Geometry: final body of the model. Coordinates: model frame, mm. A direction names the side the tool comes from. Give positions to 0.01 mm unless a question says otherwise; leave off trailing zeros. Loops run counter-clockwise (first coordinate to the right, second up) from the corner with the lowest first, then second, coordinate; pieces in that order, holes last. Notation, with made-up numbers: (-7.75, -30) -> (51.25, -30) arc R26 ccw to (51.25, -8) -> close; hole circle Ø8 at (-35, 80). An arc over 180 degrees is marked (long way). Answer in a Markdown table with one row per item. Add a question column.
from build123d import *

# Parameters (mm, degrees)
SKETCH1_W               = 50.8
SKETCH1_H               = 25.4
SKETCH1_W_2             = 44.45
SKETCH1_H_2             = 19.05
BOSS_EXTRUDE1_DEPTH     = 152.4
CUT_EXTRUDE1_DEPTH      = 163.639355631
CUT_EXTRUDE1_DEPTH_BACK = 163.639355631
SKETCH2_R               = 3.175


with BuildPart() as part:
    # Sketch1 → Boss-Extrude1 (new body)
    with BuildSketch(Plane.XY):
        with Locations((25.4, 12.7)):
            Rectangle(SKETCH1_W, SKETCH1_H)
        with Locations((25.4, 12.7)):
            Rectangle(SKETCH1_W_2, SKETCH1_H_2, mode=Mode.SUBTRACT)
    extrude(amount=BOSS_EXTRUDE1_DEPTH)

    # Sketch2 → Cut-Extrude1 (cut, two sides: drawn at the far end of the back side and taken through both)
    with BuildSketch(Plane(origin=(0, 25.4, 0), x_dir=(1, 0, 0), z_dir=(0, 1, 0)).offset(-CUT_EXTRUDE1_DEPTH_BACK)):
        with Locations(Location((12.7, -12.7, 0), (0, 0, 270))):
            Circle(SKETCH2_R)
        with Locations(Location((12.7, -50.8, 0), (0, 0, 270))):
            Circle(SKETCH2_R)
        with Locations(Location((12.7, -76.2, 0), (0, 0, 270))):
            Circle(SKETCH2_R)
        with Locations(Location((12.7, -101.6, 0), (0, 0, 270))):
            Circle(SKETCH2_R)
        with Locations(Location((12.7, -139.7, 0), (0, 0, 270))):
            Circle(SKETCH2_R)
        with Locations(Location((38.1, -139.7, 0), (0, 0, 270))):
            Circle(SKETCH2_R)
        with Locations(Location((38.1, -101.6, 0), (0, 0, 270))):
            Circle(SKETCH2_R)
        with Locations(Location((38.1, -76.2, 0), (0, 0, 270))):
            Circle(SKETCH2_R)
        with Locations(Location((38.1, -12.7, 0), (0, 0, 270))):
            Circle(SKETCH2_R)
        with Locations(Location((38.1, -50.8, 0), (0, 0, 270))):
            Circle(SKETCH2_R)
    extrude(amount=CUT_EXTRUDE1_DEPTH + CUT_EXTRUDE1_DEPTH_BACK, mode=Mode.SUBTRACT)


solid = part.part
(1) Cut plane B-B on z = 121. Return the cut outline in (x, y) (3 decimals).
(2) Pin query (flat end, axial travel): pin 1 Ø5 at (x, z) = (38.1, 139.7) entering from -Y. Return the tip coordinate at first contact, or that it passes through.
(3) Material intervals for line 1 along X through (y, z) = (24.2, 76.2) (3 decimals); line 2 along Z through (x, y) = (38.1, 24.7) (3 decimals); line 3 along Y through (x, z) = (16, 141) (3 decimals), sorted ascending. Write a range as from..to.
(4) Cut plane A-A on x = 20. Return the cut outline in (y, z) (3 decimals), then the cut area to 3 significant figures.
(5) Draft query along X for faces 1 (the flat face through (25, 23, 152.4)), 2 (the flat face through (0, 13, 75)), 3 (the cylindrical face through (12.84, 1.57, 136.53)), 4 (the flat face through (50.8, 13, 75)). Return one class per face: +X half, -X half, draft (parallel to the pull), parting line (faces both ways), or undercut.
(6) Cut plane D-D on z = 76.2. Return the cut outline in (x, y) (3 decimals), then the cut area to 3 significant figures.
(7) Cut plane C-C on y = 20.75. Return the cut outline in (x, z) (3 decimals), then the cut area to 3 significant figures.
(8) Reachability of faces 5 (the flat face through (25, 3.175, 75)), 6 (the cylindrical face through (36.17, 23.79, 10.18)) from +Z, -Z, +X, -X, +Y, -Y: full face, straight path, thin tool, end or side. Return the list, or none.
Answer list:
| question | item | result |
|---|---|---|
| 1 | outline | (0, 0) -> (50.8, 0) -> (50.8, 25.4) -> (0, 25.4) -> close; hole (3.175, 3.175) -> (47.625, 3.175) -> (47.625, 22.225) -> (3.175, 22.225) -> close |
| 2 | pin 1 | passes through |
| 3 | line 1 | x = 0..9.525, 15.875..34.925, 41.275..50.8 |
| 3 | line 2 | z = 0..9.525, 15.875..47.625, 53.975..73.025, 79.375..98.425, 104.775..136.525, 142.875..152.4 |
| 3 | line 3 | y = 0..3.175, 22.225..25.4 |
| 4 | outline | (0, 0) -> (3.175, 0) -> (3.175, 152.4) -> (0, 152.4) -> close; (22.225, 0) -> (25.4, 0) -> (25.4, 152.4) -> (22.225, 152.4) -> close |
| 4 | area | 968 mm² |
| 5 | face 1 | draft |
| 5 | face 2 | -X half |
| 5 | face 3 | undercut |
| 5 | face 4 | +X half |
| 6 | outline | (0, 0) -> (9.525, 0) -> (9.525, 3.175) -> (3.175, 3.175) -> (3.175, 22.225) -> (9.525, 22.225) -> (9.525, 25.4) -> (0, 25.4) -> close; (15.875, 0) -> (34.925, 0) -> (34.925, 3.175) -> (15.875, 3.175) -> close; (15.875, 22.225) -> (34.925, 22.225) -> (34.925, 25.4) -> (15.875, 25.4) -> close; (41.275, 0) -> (50.8, 0) -> (50.8, 25.4) -> (41.275, 25.4) -> (41.275, 22.225) -> (47.625, 22.225) -> (47.625, 3.175) -> (41.275, 3.175) -> close |
| 6 | area | 363 mm² |
| 7 | outline | (0, 0) -> (3.175, 0) -> (3.175, 152.4) -> (0, 152.4) -> close; (47.625, 0) -> (50.8, 0) -> (50.8, 152.4) -> (47.625, 152.4) -> close |
| 7 | area | 968 mm² |
| 8 | face 5 | +Z, -Z |
| 8 | face 6 | +Y, -Y |
